Part model, mm, in its own coordinate system. A direction names the side the tool comes from. Round coordinates to 2 decimals unless told otherwise and drop trailing zeros. Loops run counter-clockwise (first coordinate to the right, second up) from the corner with the lowest first, then second, coordinate; pieces in that order, holes last.
from build123d import *

# Parameters (mm, degrees)
SKETCH2_R           = 34.7138244
BOSS_EXTRUDE1_DEPTH = 43.3659661
FILLET1_R           = 2.54
SKETCH4_R           = 34.7138244
CUT_EXTRUDE1_DEPTH  = 6.985
SCALE1_SCALE        = 2.1025641


with BuildPart() as part:
    # Sketch2 → Boss-Extrude1 (new body, symmetric)
    with BuildSketch(Plane.XY):
        with Locations((-4.885886043, 8.460037767)):
            Circle(SKETCH2_R)
    extrude(amount=BOSS_EXTRUDE1_DEPTH, both=True)

    # Sketch3 → Revolve1 (revolve)
    with BuildSketch(Plane.XY):
        with BuildLine():
            Line((22.617188767, -2.954559536), (39.991940689, 15.756711766))
            ThreePointArc((39.991940689, 15.756711766), (40.875583615, 16.161668708), (41.78676132, 15.823186604))
            Line((41.78676132, 15.823186604), (42.898157249, 14.791176098))
            Line((42.898157249, 14.791176098), (48.074161234, 14.791176098))
            ThreePointArc((48.074161234, 14.791176098), (48.566620636, 14.890542194), (48.982018985, 15.173091472))
            Line((48.982018985, 15.173091472), (52.064778569, 18.324488421))
            Line((52.064778569, 18.324488421), (51.292291814, 19.080150428))
            Line((51.292291814, 19.080150428), (51.913951053, 19.715650854))
            Line((51.913951053, 19.715650854), (28.515190783, 42.604786571))
            Line((28.515190783, 42.604786571), (2.85696712, 16.37528486))
            Line((2.85696712, 16.37528486), (22.617188767, -2.954559536))
        make_face()
    revolve(axis=Axis((2.85696712, 16.37528486, 0), (0.699279233, 0.714848623, 0)))

    # Fillet1
    fillet1_edges = [part.edges().sort_by_distance(p)[0] for p in [
        (-39.599710443, 8.460037767, -43.3659661),
        (-39.599710443, 8.460037767, 43.3659661),
    ]]
    fillet(fillet1_edges, radius=FILLET1_R)

    # Sketch4 → Cut-Extrude1 (cut, symmetric)
    with BuildSketch(Plane.XY):
        with Locations((-4.885886043, 8.460037767)):
            Circle(SKETCH4_R)
    extrude(amount=CUT_EXTRUDE1_DEPTH, both=True, mode=Mode.SUBTRACT)


with BuildPart() as part_1:
    # Scale1: scaled about (0, 0, 0)
    add(part.part.scale(SCALE1_SCALE))


solid = part_1.part
1) Tool access for faces 1 (the face through (17.001, 128.983, -37.195)), 2 (the face through (-68.194, -26.624, -49.765)), 3 (the face through (-68.194, -26.624, 50.761)): list every direction of +Z, -Z, +X, -X, +Y, -Y with a clear straight run to the whole face (end or side of a thin tool).
Values:
face 1: none
face 2: -Z
face 3: +Z
2) Mould opens along Z. For faces 4 (the face through (-11, 19, 91.18)), 5 (the face through (85.76, 63.05, -58.03)), 6 (the face through (-11, 19, 14.686)) say: released by +Z, released by -Z, zero draft, split by the parting line, or undercut.
Values:
face 4: released by +Z
face 5: split by the parting line
face 6: undercut
3) Drop flat-ended pins along their axis: pin 1 Ø12 at (y, z) = (-31, -68.5) entering from +X; pin 2 Ø10 at (x, z) = (20.5, 10) entering from -Y; pin 3 Ø12 at (x, z) = (44, -44.5) entering from -Y; pin 4 Ø8 at (x, z) = (86, 68.5) entering from -Y. Give the stop position or say it passes through.
Values:
pin 1: stops at x = 48.86
pin 2: stops at y = -49.18
pin 3: stops at y = -36.96
pin 4: passes through
4) Wall check: line 1 along Z through (x, y) = (-38, 65.5); line 2 along Y through (x, z) = (25.5, -55); line 3 along Z through (x, y) = (-47, -44). Give the ranges that are in metal, low to high.
Values:
line 1: z = -91.18 to -14.69, 14.69 to 91.18
line 2: y = -45.83 to 81.41, 94.36 to 118.78
line 3: z = -89.1 to -14.69, 14.69 to 89.1
5) Slice it at A-A, the plane z = -76. Give the cut face in (x, y), then the cut area to 3 significant figures.
Values:
outline: circle Ø145.98 at (-10.27, 17.79)
area: 16,700 mm2
